The figure shows three views and two pictorial views of one solid part (mm, origin at its lowest corner). Answer the questions. A direction names the side the tool comes from. Give positions to 0.01 mm unless a question says otherwise; leave off trailing zeros. Order: outer loops, then holes, each group sorted by start corner. A loop starts at its lowest first (then second) coordinate and runs counter-clockwise, first axis right, second up. Notation, with made-up numbers: M 47,36 L 92,36 A37 ccw 92,73 Z; hole C 71.5,-10.5 d1. An arc over 180 degrees is marked long. Write item = value, one per line. Start each with the question number.
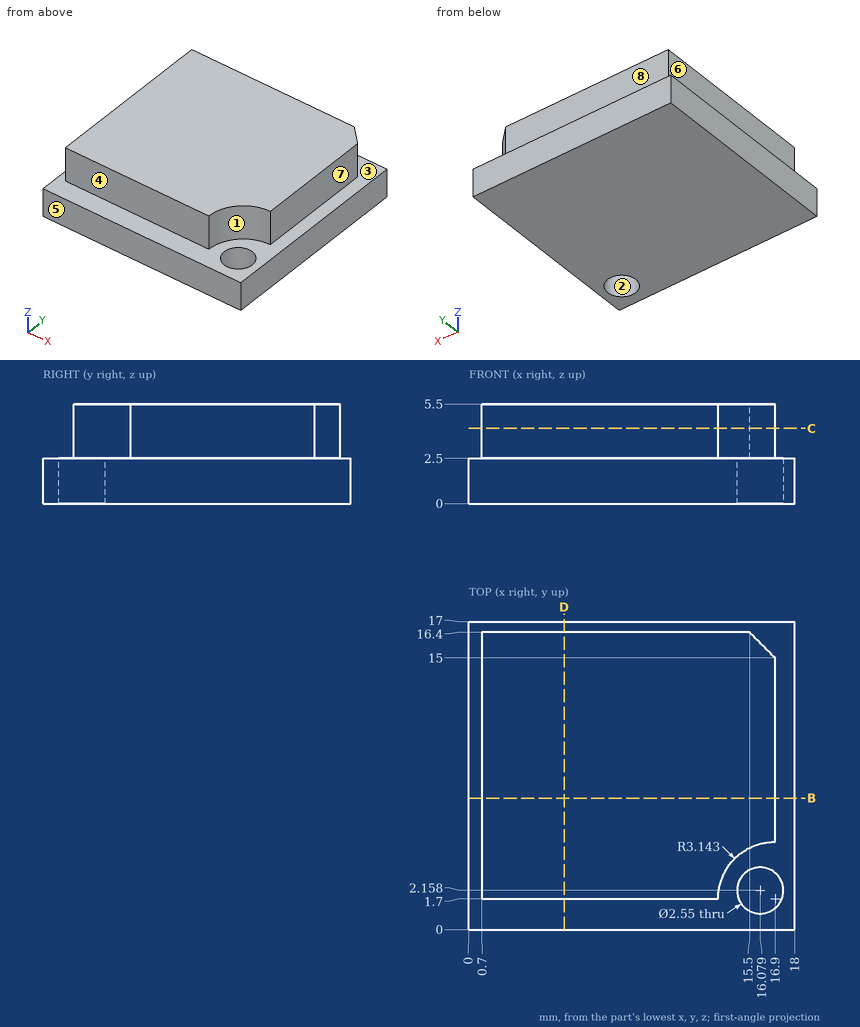
1) Find section D-D on x = 5.25. Determine the outline of the cut face in (y, z), plus the area to 3 significant figures.
2) Find section C-C on z = 4.15. Determine the outline of the cut face in (x, y) (1 decimal), plus the area to 3 significant figures.
3) Each of these flat-tipped pins is pushed along its axis until it touches: P1, Ø4, axis at x = 6, y = 5, coming from the -Z side; P2, Ø2.5, axis at y = 10, z = 4.5, coming from the +X side; P3, Ø0.9, axis at x = 10, z = 3.5, coming from the +Y side; P4, Ø1.5, axis at y = 6.5, z = 4.5, coming from the -X side. Where does it stop, or does it pass through?
4) For the marked faces 4, 5, 6, 7 and 8, determine the directions among +Z, -Z, +X, -X, +Y, -Y from which every point of the face is accessible in a straight line to the end or side of a thin tool.
5) Find the intervals of material crossed by probe 1 along Y at (x, z) = (16, 0.3) (1 decimal); probe 2 along Y at (x, z) = (3.75, 4.7); probe 3 along X at (y, z) = (13.25, 3.5), in increasing order. Write a range as [from, to].
6) Find section B-B on y = 7.25. Determine the outline of the cut face in (x, z).
7) For a pull along X with two mould halves and no side action, classify the marked faces 1, 2 and 3 as pulls with the +X half, pulls with the -X half, needs draft (parallel to the pull), parting line crosses it, or undercut.
Numbers:
q1.outline = M 0,0 L 17,0 L 17,2.5 L 16.4,2.5 L 16.4,5.5 L 1.7,5.5 L 1.7,2.5 L 0,2.5 Z
q1.area = 86.6 mm2
q2.outline = M 0.7,1.7 L 13.8,1.7 A3.1 cw 16.9,4.8 L 16.9,15 L 15.5,16.4 L 0.7,16.4 Z
q2.area = 229 mm2
q3.P1 = 0
q3.P2 = 16.9
q3.P3 = 16.4
q3.P4 = 0.7
q4.face_4 = +Z, +X, -X, -Y
q4.face_5 = +Z, -Z, +X, -X, -Y
q4.face_6 = +Z, -X, +Y, -Y
q4.face_7 = +Z, +X, +Y, -Y
q4.face_8 = +Z, +X, -X, +Y
q5.probe_1 = [0, 0.9], [3.4, 17]
q5.probe_2 = [1.7, 16.4]
q5.probe_3 = [0.7, 16.9]
q6.outline = M 0,0 L 18,0 L 18,2.5 L 16.9,2.5 L 16.9,5.5 L 0.7,5.5 L 0.7,2.5 L 0,2.5 Z
q7.face_1 = pulls with the +X half
q7.face_2 = undercut
q7.face_3 = needs draft
